```python
from build123d import *

# Parameters (mm, degrees)
SKETCH1_W           = 290
SKETCH1_H           = 50
SKETCH1_R           = 2
BOSS_EXTRUDE1_DEPTH = 4
SKETCH2_R           = 2.5
CUT_EXTRUDE1_DEPTH  = 4


with BuildPart() as part:
    # Sketch1 → Boss-Extrude1 (new body)
    with BuildSketch(Plane.XY):
        Rectangle(SKETCH1_W, SKETCH1_H)
        with Locations((-12.5, 12.5)):
            Circle(SKETCH1_R, mode=Mode.SUBTRACT)
        with Locations((12.5, 12.5)):
            Circle(SKETCH1_R, mode=Mode.SUBTRACT)
        with Locations((12.5, -12.5)):
            Circle(SKETCH1_R, mode=Mode.SUBTRACT)
        with Locations((-12.5, -12.5)):
            Circle(SKETCH1_R, mode=Mode.SUBTRACT)
    extrude(amount=BOSS_EXTRUDE1_DEPTH)

    # Sketch2 → Cut-Extrude1 (cut)
    with BuildSketch(Plane.XY.offset(4)):
        with Locations((-135, 0)):
            Circle(SKETCH2_R)
        with Locations((135, 0)):
            Circle(SKETCH2_R)
    extrude(amount=-CUT_EXTRUDE1_DEPTH, mode=Mode.SUBTRACT)


solid = part.part
```
Design review of the part built by this model. Coordinates are the model's own, in mm. Give positions to 0.01 mm unless a question says otherwise; leave off trailing zeros. Loops run counter-clockwise (first coordinate to the right, second up) from the corner with the lowest first, then second, coordinate; pieces in that order, holes last. Notation, with made-up numbers: (-28, -18) -> (-16, -18) arc R19 cw to (-16, -10) -> close; hole circle Ø9 at (38.5, 49). An arc over 180 degrees is marked (long way). One line per item, written item: value.
Q1. We need section A-A on x = -135. Give the boundary of the cut face in (y, z).
Numbers:
outline: (-25, 0) -> (-2.5, 0) -> (-2.5, 4) -> (-25, 4) -> close; (2.5, 0) -> (25, 0) -> (25, 4) -> (2.5, 4) -> close
Q2. We need section B-B on y = 0. Give the boundary of the cut face in (x, z), and give its area (3 significant figures).
Numbers:
outline: (-145, 0) -> (-137.5, 0) -> (-137.5, 4) -> (-145, 4) -> close; (-132.5, 0) -> (132.5, 0) -> (132.5, 4) -> (-132.5, 4) -> close; (137.5, 0) -> (145, 0) -> (145, 4) -> (137.5, 4) -> close
area: 1,120 mm^2
Q3. Draft analysis for pull direction X (two halves, no side actions). For faces 1 (the cylindrical face through (137.385, 0.751, 2.028)), 2 (the flat face through (-2, 0, 0)), state which applies: pulls with the +X half, pulls with the -X half, needs draft (parallel to the pull), parting line crosses it, or undercut.
Numbers:
face 1: undercut
face 2: needs draft
Q4. For L1, parallel to Y at x = 12.5, z = 2.75; L2, parallel to X at y = -11, z = 0.7; L3, parallel to X at y = 1, z = 2.9, list the stretches that pass through material, from the lowest coordinate up.
Numbers:
L1: y = -25 to -14.5, -10.5 to 10.5, 14.5 to 25
L2: x = -145 to -13.82, -11.18 to 11.18, 13.82 to 145
L3: x = -145 to -137.29, -132.71 to 132.71, 137.29 to 145
